Design review of the part built by this model. Coordinates are the model's own, in mm. A direction names the side the tool comes from. Round coordinates to 2 decimals unless told otherwise and drop trailing zeros. Loops run counter-clockwise (first coordinate to the right, second up) from the corner with the lowest first, then second, coordinate; pieces in that order, holes last. Notation, with made-up numbers: M 13,63 L 49,63 A32 cw 49,89 Z; hole C 41,33 d2. An arc over 180 degrees is marked long. Answer as CSV lines item,"result". Start each with the question number.
from build123d import *

# Parameters (mm, degrees)
SKETCH1_W           = 43
SKETCH1_H           = 43
BOSS_EXTRUDE1_DEPTH = 70
SKETCH2_R           = 20.5
CUT_EXTRUDE1_DEPTH  = 40
SKETCH3_R           = 2.25
SKETCH3_R_2         = 1.27
BOSS_EXTRUDE2_DEPTH = 4


with BuildPart() as part:
    # Sketch1 → Boss-Extrude1 (new body)
    with BuildSketch(Plane(origin=(0, 0, 0), x_dir=(1, 0, 0), z_dir=(0, 1, 0))):
        Rectangle(SKETCH1_W, SKETCH1_H)
    extrude(amount=BOSS_EXTRUDE1_DEPTH)

    # Sketch2 → Cut-Extrude1 (cut)
    with BuildSketch(Plane(origin=(21.5, 0, 0), x_dir=(0, 0, -1), z_dir=(1, 0, 0))):
        with Locations((0, 22)):
            Circle(SKETCH2_R)
    extrude(amount=-CUT_EXTRUDE1_DEPTH, mode=Mode.SUBTRACT)

    # Sketch3 → Boss-Extrude2 (add)
    # profile 1 of 4: a face of its own
    with BuildSketch(Plane(origin=(0, 70, 0), x_dir=(1, 0, 0), z_dir=(0, 1, 0))):
        with Locations(Location((17.5, 17.5, 0), (0, 0, 270))):
            Circle(SKETCH3_R)
        with Locations(Location((17.5, 17.5, 0), (0, 0, 270))):
            Circle(SKETCH3_R_2, mode=Mode.SUBTRACT)
    # profile 2 of 4: a face of its own
    with BuildSketch(Plane(origin=(0, 70, 0), x_dir=(1, 0, 0), z_dir=(0, 1, 0))):
        with Locations(Location((-17.5, 17.5, 0), (0, 0, 270))):
            Circle(SKETCH3_R)
        with Locations(Location((-17.5, 17.5, 0), (0, 0, 270))):
            Circle(SKETCH3_R_2, mode=Mode.SUBTRACT)
    # profile 3 of 4: a face of its own
    with BuildSketch(Plane(origin=(0, 70, 0), x_dir=(1, 0, 0), z_dir=(0, 1, 0))):
        with Locations(Location((-17.5, -17.5, 0), (0, 0, 270))):
            Circle(SKETCH3_R)
        with Locations(Location((-17.5, -17.5, 0), (0, 0, 270))):
            Circle(SKETCH3_R_2, mode=Mode.SUBTRACT)
    # profile 4 of 4: a face of its own
    with BuildSketch(Plane(origin=(0, 70, 0), x_dir=(1, 0, 0), z_dir=(0, 1, 0))):
        with Locations(Location((17.5, -17.5, 0), (0, 0, 270))):
            Circle(SKETCH3_R)
        with Locations(Location((17.5, -17.5, 0), (0, 0, 270))):
            Circle(SKETCH3_R_2, mode=Mode.SUBTRACT)
    extrude(amount=BOSS_EXTRUDE2_DEPTH)


solid = part.part
Item 1: Consider section D-D, the plane x = -1. Write out the cut boundary in (y, z), then the cut area to 3 significant figures.
Item 2: Consider section C-C, the plane y = 36. Write out the cut boundary in (x, z).
Item 3: The part is to be moulded in two halves that separate along X. For faces 4 (the face through (-18, 70, -18)), 5 (the face through (-21.5, 35, 0)), 6 (the face through (-19, 74, -18)), say which applies: +X half, -X half, draft (parallel to the pull), parting line (faces both ways), or undercut.
Item 4: Tool access review of faces 1 (the face through (0, 35, 21.5)), 2 (the face through (0, 70, 0)), 3 (the face through (1.78, 28.158, -19.553)): name each direction out of +Z, -Z, +X, -X, +Y, -Y from which nothing blocks a thin tool from reaching the whole face with its end or side.
Item 5: Insertion check: pin 1 Ø12.5 at (y, z) = (19.5, 0) entering from +X; pin 2 Ø0.8 at (x, z) = (-17.5, 18) entering from +Y. Each pin has a flat end and moves straight along its axis. Give the tip position at first contact, or say it passes through.
Item 6: Consider section B-B, the plane z = 0. Write out the cut boundary in (x, y), then the cut area to 3 significant figures.
Item 7: Consider section A-A, the plane x = -17.5. Write out the cut boundary in (y, z), then the cut area to 3 significant figures.
Item 8: To check wall thickness, follow line 1 (X direction, y = 72.8, z = 17.5); line 2 (Z direction, x = -17, y = 71); line 3 (X direction, y = 38, z = 12). State the ranges of each line that lie inside material, in increasing order.
Found:
1,outline,"M 0,-21.5 L 70,-21.5 L 70,21.5 L 0,21.5 Z; hole C 22,0 d41"
1,area,"1,690 mm^2"
2,outline,"M -21.5,-21.5 L 21.5,-21.5 L 21.5,-14.97 L -18.5,-14.97 L -18.5,14.97 L 21.5,14.97 L 21.5,21.5 L -21.5,21.5 Z"
3,face 4,"undercut"
3,face 5,"-X half"
3,face 6,"draft"
4,face 1,"+Z, +X, -X, +Y, -Y"
4,face 2,"+Y"
4,face 3,"+X"
5,pin 1,"stops at x = -18.5"
5,pin 2,"stops at y = 70"
6,outline,"M -21.5,0 L 21.5,0 L 21.5,1.5 L -18.5,1.5 L -18.5,42.5 L 21.5,42.5 L 21.5,70 L -21.5,70 Z"
6,area,"1,370 mm^2"
7,outline,"M 0,-21.5 L 70,-21.5 L 70,-19.75 L 74,-19.75 L 74,-18.77 L 70,-18.77 L 70,-16.23 L 74,-16.23 L 74,-15.25 L 70,-15.25 L 70,15.25 L 74,15.25 L 74,16.23 L 70,16.23 L 70,18.77 L 74,18.77 L 74,19.75 L 70,19.75 L 70,21.5 L 0,21.5 Z; hole C 22,0 d41"
7,area,"1,710 mm^2"
8,line 1,"x = -19.75 to -18.77, -16.23 to -15.25, 15.25 to 16.23, 18.77 to 19.75"
8,line 2,"z = -19.69 to -18.67, -16.33 to -15.31, 15.31 to 16.33, 18.67 to 19.69"
8,line 3,"x = -21.5 to -18.5"
